Input: part model. Units: mm. Frame: model coordinates. A direction names the side the tool comes from. Coordinates: 2 decimals unless noted, no trailing zeros. Loops run counter-clockwise (first coordinate to the right, second up) from the corner with the lowest first, then second, coordinate; pieces in that order, holes last. Notation, with made-up numbers: (52, -5.75) - (75, -5.75) arc R27 ccw to (75, 13.25) - close; hole circle Ø8 at (40.25, -21). An arc over 180 degrees is marked (long way). Use a Markdown table: item, result. Add a question column.
1. Section query B-B on x = -5. Return the cut outline in (y, z) (3 decimals).
2. Contact query for flat-ended pins moving along their axis: P1, Ø2, axis at x = 8, z = 0, coming from the +Y side (3 decimals); P2, Ø2.5, axis at x = 10, y = 17, coming from the +Z side; P3, Ø11, axis at x = 3, z = 5.5, coming from the -Y side; P4, Ø5, axis at x = 12, z = -1.5, coming from the +Y side. Output: stop coordinate, or through.
3. Ray query, L1, parallel to X at y = 8.25, z = 0; L2, parallel to Z at x = -19, y = 14.5; L3, parallel to Y at x = -10.5, z = -8.25. Return the intervals inside material, ascending. Write a range as [from, to].
4. Access query for faces 1 (the face through (9, 17, -3.175)), 2 (the face through (16, 9, 6.223)), 3 (the face through (9.5, 9.219, -11.754)), 4 (the face through (-3, 12, -12)), 5 (the face through (-20.806, -4.829, -1.346)). Directions: +Z, -Z, +X, -X, +Y, -Y. A direction counts if a zero-diameter tool reaches every point of the face in a straight line with its end or side. Return the directions, or none.
5. Section query C-C on y = 9.25. Return the cut outline in (x, z).
6. Section query A-A on z = 7. Return the cut outline in (x, y), then the cut area to 3 significant figures.
7. Draft query along X for faces 6 (the face through (-9.34, 9.22, -11.88)), 7 (the face through (11, 15.525, 0)), 8 (the face through (-16, 9, 6.223)). Return one class per face: released by +X, released by -X, zero draft, split by the parting line, or undercut.
8. Section query D-D on z = 13. Return the cut outline in (x, y).
```python
from build123d import *

# Parameters (mm, degrees)
SKETCH1_R             = 11.303
BOSS_EXTRUDE1_DEPTH   = 12.7
F_4_40_TAPPED_HOLE1_D = 2.2606
SKETCH10_R            = 2.38125
BOSS_EXTRUDE2_DEPTH   = 9.525
BOSS_EXTRUDE2_TAPER   = 2
SKETCH14_R            = 11.303
SKETCH14_R_2          = 8
BOSS_EXTRUDE3_DEPTH   = 6
SKETCH20_W            = 6
SKETCH20_H            = 15.993334041
CUT_EXTRUDE3_DEPTH    = 29.2250001
CUT_EXTRUDE4_DEPTH    = 3.175


with BuildPart() as part:
    # Sketch1 → Boss-Extrude1 (new body)
    with BuildSketch(Plane(origin=(0, 0, 0), x_dir=(1, 0, 0), z_dir=(0, 1, 0))):
        with BuildLine():
            Line((-19.05, 6.223), (-13.772328779, 6.223))
            ThreePointArc((-13.772328779, 6.223), (0, 15.113), (13.772328779, 6.223))
            Line((13.772328779, 6.223), (19.05, 6.223))
            ThreePointArc((19.05, 6.223), (25.273, 0), (19.05, -6.223))
            Line((19.05, -6.223), (13.772328779, -6.223))
            ThreePointArc((13.772328779, -6.223), (0, -15.113), (-13.772328779, -6.223))
            Line((-13.772328779, -6.223), (-19.05, -6.223))
            ThreePointArc((-19.05, -6.223), (-25.273, 0), (-19.05, 6.223))
        make_face()
        Circle(SKETCH1_R, mode=Mode.SUBTRACT)
    extrude(amount=BOSS_EXTRUDE1_DEPTH)

    # #4-40 Tapped Hole1 (through all)
    with Locations(Plane.XY.offset(15.113)):
        with Locations((0, 2.38125)):
            Hole(F_4_40_TAPPED_HOLE1_D / 2)

    # Sketch10 → Boss-Extrude2 (add)
    with BuildSketch(Plane.XZ):
        with Locations((-19.05, 0)):
            Circle(SKETCH10_R)
        with Locations((19.05, 0)):
            Circle(SKETCH10_R)
    extrude(amount=BOSS_EXTRUDE2_DEPTH, taper=BOSS_EXTRUDE2_TAPER)

    # Sketch14 → Boss-Extrude3 (add)
    with BuildSketch(Plane(origin=(0, 12.7, 0), x_dir=(1, 0, 0), z_dir=(0, 1, 0))):
        with BuildLine():
            ThreePointArc((13.772328779, 6.223), (14.774030828, 3.182888952), (15.113, 0))
            ThreePointArc((15.113, 0), (14.774030828, -3.182888952), (13.772328779, -6.223))
            Line((13.772328779, -6.223), (19.05, -6.223))
            ThreePointArc((19.05, -6.223), (25.273, 0), (19.05, 6.223))
            Line((19.05, 6.223), (13.772328779, 6.223))
        make_face()
        with BuildLine():
            ThreePointArc((-13.772328779, -6.223), (-15.113, 0), (-13.772328779, 6.223))
            Line((-13.772328779, 6.223), (-19.05, 6.223))
            ThreePointArc((-19.05, 6.223), (-25.273, 0), (-19.05, -6.223))
            Line((-19.05, -6.223), (-13.772328779, -6.223))
        make_face()
        with BuildLine():
            ThreePointArc((13.772328779, -6.223), (14.774030828, -3.182888952), (15.113, 0))
            ThreePointArc((15.113, 0), (14.774030828, 3.182888952), (13.772328779, 6.223))
            ThreePointArc((13.772328779, 6.223), (0, 15.113), (-13.772328779, 6.223))
            ThreePointArc((-13.772328779, 6.223), (-15.113, 0), (-13.772328779, -6.223))
            ThreePointArc((-13.772328779, -6.223), (0, -15.113), (13.772328779, -6.223))
        make_face()
        Circle(SKETCH14_R, mode=Mode.SUBTRACT)
        Circle(SKETCH14_R)
        Circle(SKETCH14_R_2, mode=Mode.SUBTRACT)
    extrude(amount=BOSS_EXTRUDE3_DEPTH)

    # Sketch20 → Cut-Extrude3 (cut, through all)
    with BuildSketch(Plane(origin=(0, 18.7, 0), x_dir=(1, 0, 0), z_dir=(0, 1, 0))):
        with Locations((0, 10.151613004)):
            Rectangle(SKETCH20_W, SKETCH20_H)
    extrude(amount=-CUT_EXTRUDE3_DEPTH, mode=Mode.SUBTRACT)

    # Sketch21 → Cut-Extrude4 (cut)
    with BuildSketch(Plane(origin=(0, 18.7, 0), x_dir=(1, 0, 0), z_dir=(0, 1, 0))):
        with BuildLine():
            Line((-10.700000063, 3.175), (10.700000063, 3.175))
            ThreePointArc((10.700000063, 3.175), (13.875000063, 0), (10.700000063, -3.175))
            Line((10.700000063, -3.175), (-10.700000063, -3.175))
            ThreePointArc((-10.700000063, -3.175), (-13.875000063, 0), (-10.700000063, 3.175))
        make_face()
    extrude(amount=-CUT_EXTRUDE4_DEPTH, mode=Mode.SUBTRACT)


solid = part.part
```
Resolved:
| question | item | result |
|---|---|---|
| 1 | outline | (0, -14.262) - (18.7, -14.262) - (18.7, -6.245) - (12.7, -6.245) - (12.7, -10.137) - (0, -10.137) - close; (0, 10.137) - (12.7, 10.137) - (12.7, 6.245) - (18.7, 6.245) - (18.7, 14.262) - (0, 14.262) - close |
| 2 | P1 | y = 15.525 |
| 2 | P2 | z = 12.32 |
| 2 | P3 | y = 0 |
| 2 | P4 | y = 18.7 |
| 3 | L1 | [-25.27, -11.3], [11.3, 25.27] |
| 3 | L2 | [-6.22, 6.22] |
| 3 | L3 | [0, 18.7] |
| 4 | face 1 | +Y |
| 4 | face 2 | +Z, +X, +Y, -Y |
| 4 | face 3 | -Z, +X, +Y, -Y |
| 4 | face 4 | -Z, +Y, -Y |
| 4 | face 5 | -Y |
| 5 | outline | (-19.05, -6.22) - (-13.77, -6.22) arc R15.11 ccw to (-3, -14.81) - (-3, -10.9) arc R11.3 cw (long way) to (3, -10.9) - (3, -14.81) arc R15.11 ccw to (13.77, -6.22) - (19.05, -6.22) arc R6.22 ccw to (19.05, 6.22) - (13.77, 6.22) arc R15.11 ccw to (-13.77, 6.22) - (-19.05, 6.22) arc R6.22 ccw to start |
| 6 | outline | (-13.39, 0) - (-8.87, 0) - (-8.87, 12.7) - (-3.87, 12.7) - (-3.87, 18.7) - (-13.39, 18.7) - close; (3.87, 12.7) - (8.87, 12.7) - (8.87, 0) - (13.39, 0) - (13.39, 18.7) - (3.87, 18.7) - close |
| 6 | area | 229 mm² |
| 7 | face 6 | released by -X |
| 7 | face 7 | undercut |
| 7 | face 8 | zero draft |
| 8 | outline | (-7.71, 0) - (7.71, 0) - (7.71, 18.7) - (-7.71, 18.7) - close; hole circle Ø2.26 at (0, 2.38) |
